Source: three-view drawing plus pictorial views. Frame: mm from the lowest corner of the part. A direction names the side the tool comes from. Give positions to 0.01 mm unless a question says otherwise; leave off trailing zeros. Write each loop counter-clockwise with the first axis right and the second up, starting at its lowest first coordinate (ties: lowest second). Pieces come first, ordered by that corner, then holes. Notation, with made-up numbers: (26.5, 56.25) -> (42.5, 56.25) arc R26 cw to (42.5, 93.25) -> close; hole circle Ø8 at (63.5, 46.5). An arc over 180 degrees is marked (long way). Write item = value, one per line.
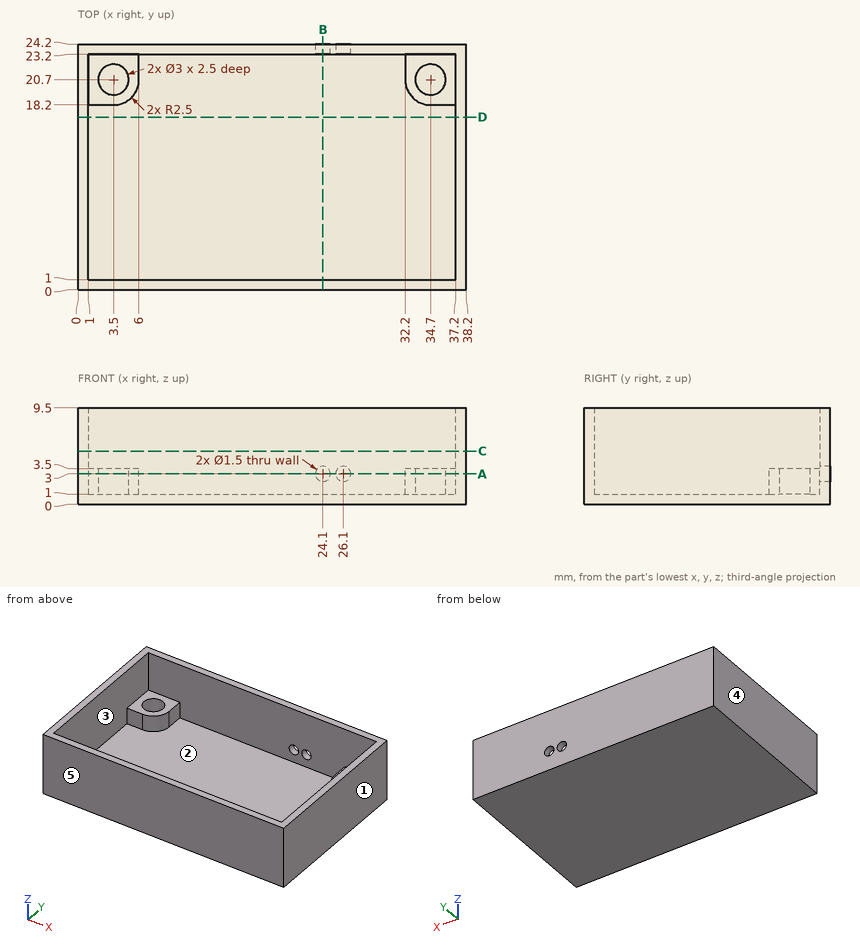
1) Cut plane A-A (z = 3). Return the cut outline in (x, y).
Computed:
outline = (0, 0) -> (38.2, 0) -> (38.2, 24.2) -> (26.85, 24.2) -> (26.85, 23.2) -> (32.2, 23.2) -> (32.2, 20.7) arc R2.5 ccw to (34.7, 18.2) -> (37.2, 18.2) -> (37.2, 1) -> (1, 1) -> (1, 18.2) -> (3.5, 18.2) arc R2.5 ccw to (6, 20.7) -> (6, 23.2) -> (23.35, 23.2) -> (23.35, 24.2) -> (0, 24.2) -> close; (24.85, 23.2) -> (25.35, 23.2) -> (25.35, 24.2) -> (24.85, 24.2) -> close; hole circle Ø3 at (3.5, 20.7); hole circle Ø3 at (34.7, 20.7)
2) Draft query along X for the marked faces 3, 4 and 5. Return one class per face: pulls with the +X half, pulls with the -X half, needs draft (parallel to the pull), parting line crosses it, or undercut.
Computed:
face_3 = undercut
face_4 = pulls with the -X half
face_5 = needs draft
3) Access query for the marked faces 1 and 2. Directions: +Z, -Z, +X, -X, +Y, -Y. A direction counts if a zero-diameter tool reaches every point of the face in a straight line with its end or side. Return the directions, or none.
Computed:
face_1 = +Z, -Z, +X, +Y, -Y
face_2 = +Z
4) Contact query for flat-ended pins moving along their axis: pin 1 (1.5 mm diameter, centred on x = 34, y = 21.5, fed in from +Z); pin 2 (1.5 mm diameter, centred on x = 3, y = 20.5, fed in from +Z). Output: stop coordinate, or through.
Computed:
pin_1 = 3.5
pin_2 = 1
5) Material intervals for L1, parallel to X at y = 10.75, z = 7.75; L2, parallel to Y at x = 19.5, z = 6; L3, parallel to Z at x = 26.1, y = 23.5, sorted ascending.
Computed:
L1 = 0 to 1, 37.2 to 38.2
L2 = 0 to 1, 23.2 to 24.2
L3 = 0 to 2.25, 3.75 to 9.5
6) Cut plane C-C (z = 5.25). Return the cut outline in (x, y), then the cut area to 3 significant figures.
Computed:
outline = (0, 0) -> (38.2, 0) -> (38.2, 24.2) -> (0, 24.2) -> close; hole (1, 1) -> (37.2, 1) -> (37.2, 23.2) -> (1, 23.2) -> close
area = 121 mm²
7) Cut plane D-D (y = 17). Return the cut outline in (x, z).
Computed:
outline = (0, 0) -> (38.2, 0) -> (38.2, 9.5) -> (37.2, 9.5) -> (37.2, 1) -> (1, 1) -> (1, 9.5) -> (0, 9.5) -> close
8) Cut plane B-B (x = 24.1). Return the cut outline in (y, z).
Computed:
outline = (0, 0) -> (24.2, 0) -> (24.2, 2.25) -> (23.2, 2.25) -> (23.2, 1) -> (1, 1) -> (1, 9.5) -> (0, 9.5) -> close; (23.2, 3.75) -> (24.2, 3.75) -> (24.2, 9.5) -> (23.2, 9.5) -> close
